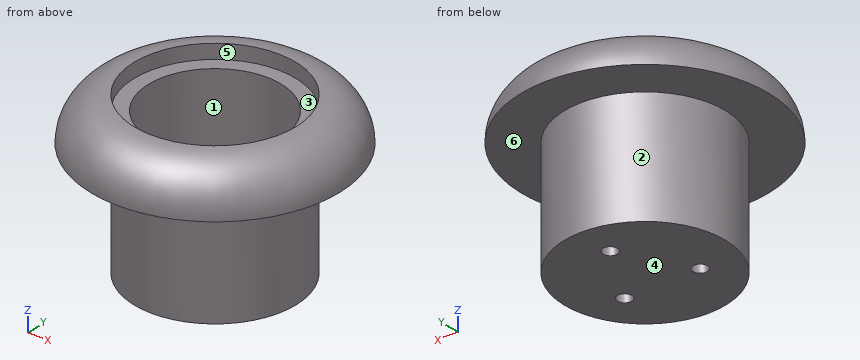
```python
from build123d import *

# Parameters (mm, degrees)
F2_R     = 14.99999
F4_D     = 5
F5_R     = 28
F5_R_2   = 23
F6_DEPTH = 5


# Not quite as in the source:
# - a fillet or chamfer is up to 0.001 mm smaller than in the source, because OpenCascade refuses the exact size


with BuildPart() as f1:
    # F0 (on Front) → F1 (revolve)
    with BuildSketch(Plane.XZ):
        Polygon((43, 15), (43, 30), (23, 30), (23, -20), (0, -20), (0, -25), (28, -25), (28, -15), (28, 15), align=None)
    revolve(axis=Axis((0, 0, -22.5), (0, 0, -1)))

    # F2 (radius 15 in the source; OpenCascade refuses exactly that, so slightly less here)
    f2_edges = [f1.edges().sort_by_distance(p)[0] for p in [
        (-43, 0, 30),
    ]]
    fillet(f2_edges, radius=F2_R)

    # F4 (through all)
    with Locations(Plane.XY.offset(-20)):
        with Locations((0, 15), (-12.9903810568, -7.5), (12.9903810568, -7.5)):
            Hole(F4_D / 2)

    # F5 (on face) → F6 (cut)
    with BuildSketch(Plane.XY.offset(30)):
        Circle(F5_R)
        Circle(F5_R_2, mode=Mode.SUBTRACT)
    extrude(amount=-F6_DEPTH, mode=Mode.SUBTRACT)


solid = f1.part
```
Here's how the part is built. I have some questions about the finished solid (model axes, mm). Face numbers are marked on the shaded views. A direction names the side the tool comes from. Round coordinates to 2 decimals unless told otherwise and drop trailing zeros. Write each loop counter-clockwise with the first axis right and the second up, starting at its lowest first coordinate (ties: lowest second). Pieces come first, ordered by that corner, then holes.
Q1. Which directions (+Z, -Z, +X, -X, +Y, -Y) give clear straight access to the entire face, cutting with the end or side of a thin tool? Please do the marked faces 5 and 6.
Q2. If we section it at C-C on z = -8: Write out the boundary of the cut face in (x, y), plus the area to 3 significant figures.
Q3. If we mould it in two halves opening along X, with no side actions, what happens to the marked faces 1, 2, 3 and 4? For each: +X half, -X half, draft (parallel to the pull), parting line (faces both ways), or undercut.
Q4. Please list where these lines run through material, in increasing order: probe 1 along Y at (x, z) = (0, 2); probe 2 along Y at (x, z) = (24.5, 27); probe 3 along X at (y, z) = (11.5, 27.5).
Q5. Will these pins go through, and if not, where does the flat tip stop? P1, Ø3, axis at x = -17.5, y = 27.5, coming from the -Z side; P2, Ø3, axis at x = -3, z = -16, coming from the -Y side; P3, Ø12, axis at x = 19.5, y = -1.5, coming from the +Z side; P4, Ø4.5, axis at x = 0, y = 15, coming from the -Z side.
Answer below:
1. face 5: +Z
1. face 6: -Z
2. outline: circle Ø56 at (0, 0); hole circle Ø46 at (0, 0)
2. area: 801 mm2
3. face 1: undercut
3. face 2: parting line
3. face 3: undercut
3. face 4: draft
4. probe 1: y = -28 to -23, 23 to 28
4. probe 2: y = -27.73 to -13.56, 13.56 to 27.73
4. probe 3: x = -34.42 to -25.53, 25.53 to 34.42
5. P1: stops at z = 15
5. P2: stops at y = -27.96
5. P3: stops at z = 25
5. P4: passes through
